```python
from build123d import *

# Parameters (mm, degrees)
F0_R     = 73.025
F0_R_2   = 2.54
F0_R_3   = 3.175
F1_DEPTH = 1.27
F2_W     = 11.43
F2_H     = 36.83
F3_DEPTH = 1.271


with BuildPart() as f1:
    # F0 (on Top) → F1 (new body)
    with BuildSketch(Plane.XY):
        Circle(F0_R)
        with Locations((0, -69.215)):
            Circle(F0_R_2, mode=Mode.SUBTRACT)
        with Locations((-69.215, 0)):
            Circle(F0_R_2, mode=Mode.SUBTRACT)
        Circle(F0_R_3, mode=Mode.SUBTRACT)
        with Locations((69.215, 0)):
            Circle(F0_R_2, mode=Mode.SUBTRACT)
        with Locations((0, 69.215)):
            Circle(F0_R_2, mode=Mode.SUBTRACT)
    extrude(amount=F1_DEPTH)

    # F2 (on face) → F3 (cut, through all)
    with BuildSketch(Plane.XY.offset(1.27)):
        with Locations((-59.69, 0)):
            Rectangle(F2_W, F2_H)
        with Locations((59.69, 0)):
            Rectangle(F2_W, F2_H)
    extrude(amount=-F3_DEPTH, mode=Mode.SUBTRACT)


solid = f1.part
```
CAD build for the part. Positions are in the model's coordinates, mm. Give positions to 0.01 mm unless a question says otherwise; leave off trailing zeros. Loops run counter-clockwise (first coordinate to the right, second up) from the corner with the lowest first, then second, coordinate; pieces in that order, holes last. Notation, with made-up numbers: (42, 22) - (58, 22) arc R21 ccw to (58, 34) - close; hole circle Ø5 at (-10, -9.75). An arc over 180 degrees is marked (long way). Put each result on its own line as item: value.
Q1. Slice it at A-A (y = 0). Give the cut face in (x, z) (3 decimals), plus the area to 3 significant figures.
Filled in:
outline: (-73.025, 0) - (-71.755, 0) - (-71.755, 1.27) - (-73.025, 1.27) - close; (-66.675, 0) - (-65.405, 0) - (-65.405, 1.27) - (-66.675, 1.27) - close; (-53.975, 0) - (-3.175, 0) - (-3.175, 1.27) - (-53.975, 1.27) - close; (3.175, 0) - (53.975, 0) - (53.975, 1.27) - (3.175, 1.27) - close; (65.405, 0) - (66.675, 0) - (66.675, 1.27) - (65.405, 1.27) - close; (71.755, 0) - (73.025, 0) - (73.025, 1.27) - (71.755, 1.27) - close
area: 135 mm²
Q2. Slice it at B-B (x = 0). Give the cut face in (y, z) (3 decimals), plus the area to 3 significant figures.
Filled in:
outline: (-73.025, 0) - (-71.755, 0) - (-71.755, 1.27) - (-73.025, 1.27) - close; (-66.675, 0) - (-3.175, 0) - (-3.175, 1.27) - (-66.675, 1.27) - close; (3.175, 0) - (66.675, 0) - (66.675, 1.27) - (3.175, 1.27) - close; (71.755, 0) - (73.025, 0) - (73.025, 1.27) - (71.755, 1.27) - close
area: 165 mm²
Q3. Slice it at C-C (z = 0.25). Give the cut face in (x, y) (3 decimals).
Filled in:
outline: circle Ø146.05 at (0, 0); hole circle Ø5.08 at (-69.215, 0); hole (-65.405, -18.415) - (-53.975, -18.415) - (-53.975, 18.415) - (-65.405, 18.415) - close; hole circle Ø6.35 at (0, 0); hole circle Ø5.08 at (0, -69.215); hole circle Ø5.08 at (0, 69.215); hole (53.975, -18.415) - (65.405, -18.415) - (65.405, 18.415) - (53.975, 18.415) - close; hole circle Ø5.08 at (69.215, 0)
Q4. Probe line 1 along Y through (x, z) = (0, 0.7) (3 decimals); line 2 along X through (y, z) = (13, 0.65) (3 decimals); line 3 along X through (y, z) = (7.5, 0.85) (3 decimals). List the from-to ranges inside material, lowest first.
Filled in:
line 1: y = -73.025 to -71.755, -66.675 to -3.175, 3.175 to 66.675, 71.755 to 73.025
line 2: x = -71.859 to -65.405, -53.975 to 53.975, 65.405 to 71.859
line 3: x = -72.639 to -65.405, -53.975 to 53.975, 65.405 to 72.639
Q5. Flat gauge pins, fed straight in: pin 1 (0.6 mm diameter, centred on y = -7.5, z = 1, fed in from +X); pin 2 (7.5 mm diameter, centred on x = 0, y = 0, fed in from -Z). Where does each tip first touch, or does it go through?
Filled in:
pin 1: stops at x = 72.67
pin 2: stops at z = 0
Q6. Slice it at D-D (y = 34). Give the cut face in (x, z).
Filled in:
outline: (-64.63, 0) - (64.63, 0) - (64.63, 1.27) - (-64.63, 1.27) - close
Q7. Mould opens along Y. For faces 1 (the face through (66.677, 0.112, 0.626)), 2 (the face through (69.653, 21.935, 0.626)), 3 (the face through (-0.331, 71.733, 0.626)), 4 (the face through (-1, -15, 0)) say: pulls with the +Y half, pulls with the -Y half, needs draft (parallel to the pull), parting line crosses it, or undercut.
Filled in:
face 1: undercut
face 2: parting line crosses it
face 3: undercut
face 4: needs draft
